from build123d import *

# Parameters (mm, degrees)
F0_W     = 50.8
F0_H     = 31.75
F1_DEPTH = 25.4
F3_DEPTH = 31.75
F4_W     = 19.05
F4_H     = 19.05
F5_DEPTH = 19.05


with BuildPart() as f1:
    # F0 (on Top) → F1 (new body)
    with BuildSketch(Plane.XY):
        with Locations((25.4, 15.875)):
            Rectangle(F0_W, F0_H)
    extrude(amount=F1_DEPTH)

    # F2 (on face) → F3 (cut)
    with BuildSketch(Plane.XZ):
        Polygon((19.05, 25.4), (50.8, 0), (50.8, 25.4), align=None)
    extrude(amount=-F3_DEPTH, mode=Mode.SUBTRACT)

    # F4 (on face) → F5 (join)
    with BuildSketch(Plane(origin=(0, 0, 0), x_dir=(1, 0, 0), z_dir=(0, 0, -1))):
        with Locations((41.275, -22.225)):
            Rectangle(F4_W, F4_H)
    extrude(amount=-F5_DEPTH)


solid = f1.part
Here's how the part is built. I have some questions about the finished solid (model axes, mm). A direction names the side the tool comes from. Coordinates: 2 decimals unless noted, no trailing zeros. Order: outer loops, then holes, each group sorted by start corner. A loop starts at its lowest first (then second) coordinate and runs counter-clockwise, first axis right, second up. Notation, with made-up numbers: (-23, 55) - (27, 55) arc R20 cw to (27, 62) - close; hole circle Ø9 at (85.5, 33.25). An arc over 180 degrees is marked (long way). Use CSV: the item, a comma, the result in double quotes. Start each with the question number.
1. Please list where these lines run through material, in increasing order: line 1 (Z direction, x = 45, y = 26.5); line 2 (Y direction, x = 39, z = 11); line 3 (Z direction, x = 23, y = 18.5). Write a range as from..to.
2. Suppose I cut it at D-D on z = 21. List the corners of the cut face in (x, y) for me.
3. Suppose I cut it at B-B on y = 25. List the corners of the cut face in (x, z) for me.
4. I'm going to push flat-ended pins straight in: pin 1 (6 mm diameter, centred on y = 9, z = 14.5, fed in from +X) (3 decimals); pin 2 (9.5 mm diameter, centred on x = 43.5, y = 18.5, fed in from +Z). Where does each tip first touch, or does it pass through?
5. Suppose I cut it at C-C on x = 24. List the corners of the cut face in (y, z) for me.
6. If we mould it in two halves opening along X, with no side actions, what happens to faces 3 (the face through (41, 22, 19.05)), 4 (the face through (31.75, 22, 17)), 5 (the face through (50.8, 22, 9))? For each: +X half, -X half, draft (parallel to the pull), parting line (faces both ways), or undercut.
7. Suppose I cut it at A-A on z = 17. List the corners of the cut face in (x, y) for me.
8. For faces 1 (the face through (43, 12.7, 12)), 2 (the face through (19, 0, 10)), which set-ups out of +Z, -Z, +X, -X, +Y, -Y let a thin tool reach every point of the face, with its end or its side?
Output:
1,line 1,"z = 0..19.05"
1,line 2,"y = 12.7..31.75"
1,line 3,"z = 0..22.24"
2,outline,"(0, 0) - (24.55, 0) - (24.55, 31.75) - (0, 31.75) - close"
3,outline,"(0, 0) - (50.8, 0) - (50.8, 19.05) - (31.75, 19.05) - (31.75, 15.24) - (19.05, 25.4) - (0, 25.4) - close"
4,pin 1,"stops at x = 36.425"
4,pin 2,"stops at z = 19.05"
5,outline,"(0, 0) - (31.75, 0) - (31.75, 21.44) - (0, 21.44) - close"
6,face 3,"draft"
6,face 4,"undercut"
6,face 5,"+X half"
7,outline,"(0, 0) - (29.55, 0) - (29.55, 31.75) - (0, 31.75) - close; (31.75, 12.7) - (50.8, 12.7) - (50.8, 31.75) - (31.75, 31.75) - close"
8,face 1,"+Z, +X, -Y"
8,face 2,"+Z, -Z, +X, -X, -Y"
